Input: part model. Units: mm. Frame: model coordinates. Coordinates: 2 decimals unless noted, no trailing zeros. Write each loop counter-clockwise with the first axis right and the second up, starting at its lowest first coordinate (ties: lowest second). Pieces come first, ordered by that corner, then holes. Notation, with made-up numbers: (-17.5, 81) -> (22.5, 81) arc R27 ccw to (22.5, 119) -> close; hole circle Ø8 at (-26.5, -23). An arc over 180 degrees is marked (long way). One line per question, with ' | ' between items. Start each with the question number.
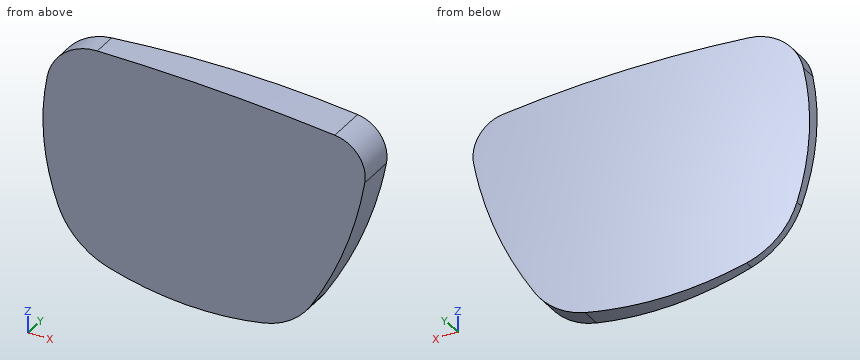
```python
from build123d import *

# Parameters (mm, degrees)
F1_DEPTH      = 25
F4_ANGLE_BACK = 15
F4_ANGLE      = 30


with BuildPart() as f1:
    # F0 (on Front) → F1 (new body)
    with BuildSketch(Plane.XZ):
        with BuildLine():
            ThreePointArc((26.3431364877, 8.5707053028), (25.1879544986, 13.2060879092), (21.0133194591, 15.5285089783))
            ThreePointArc((21.0133194591, 15.5285089783), (-0.0894086287, 17.0460813995), (-21.2428583947, 17.4457334904))
            ThreePointArc((-21.2428583947, 17.4457334904), (-27.0252643869, 15.3277245971), (-30.1521339791, 10.0225509634))
            ThreePointArc((-30.1521339791, 10.0225509634), (-30.737948683, -1.5598670025), (-28.1338702514, -12.8609448416))
            ThreePointArc((-28.1338702514, -12.8609448416), (-24.6579753008, -18.0246958087), (-19.2665178824, -21.1357015406))
            ThreePointArc((-19.2665178824, -21.1357015406), (-5.5690318774, -23.5254263951), (8.2977543738, -22.503591381))
            ThreePointArc((8.2977543738, -22.503591381), (13.1377213939, -20.4559972218), (16.7715565718, -16.6595298512))
            ThreePointArc((16.7715565718, -16.6595298512), (22.8064529235, -4.5182850542), (26.3431364877, 8.5707053028))
        make_face()
    extrude(amount=-F1_DEPTH)


with BuildPart() as f4:
    # F3 (on offset) → F4 (revolve)
    with BuildSketch(Plane.XY.offset(22), mode=Mode.PRIVATE) as f4_sk:
        with BuildLine():
            Line((-282, -293), (318, -293))
            ThreePointArc((318, -293), (18, 7), (-282, -293))
        make_face()
    revolve(f4_sk.sketch.rotate(Axis((18, -293, 22), (1, 0, 0)), -F4_ANGLE_BACK), axis=Axis((18, -293, 22), (1, 0, 0)), revolution_arc=F4_ANGLE)


with BuildPart() as f1_1:
    add(f1.part)

    # F5: intersect F4
    add(f4.part, mode=Mode.INTERSECT)


solid = f1_1.part
```
1) Section A-A, the plane y = 2.25. Return loops of the section in (x, z) (1 decimal).
2) Ray query, line 1 (Z direction, x = 20.5, y = 1.25); line 2 (Y direction, x = 2, z = 7); line 3 (Z direction, x = 18, y = 3.25). Return the intervals inside material, ascending.
3) First-contact query: P1, Ø6, axis at x = -24.5, z = -0.5, coming from the +Y side; P2, Ø4, axis at x = 6, y = 1, coming from the -Z side; P3, Ø1.5, axis at x = -24.5, z = -17, coming from the -Y side; P4, Ø1.5, axis at y = 2.5, z = 6, coming from the -X side. Flat tips, straight axial feed; report the tip coordinate or a pass-through.
4) Section B-B, the plane z = 14. Return loops of the section in (x, y), then the cut area to 3 significant figures.
5) Section C-C, the plane x = -16.5. Return loops of the section in (y, z).
Answer block:
1) outline: (-30.9, 1.1) arc R53.2 ccw to (-10.2, -23.1) arc R56.6 ccw to (8.3, -22.5) arc R13 ccw to (16.8, -16.7) arc R68.8 ccw to (26.3, 8.6) arc R6 ccw to (21, 15.5) arc R400 ccw to (-21.2, 17.4) arc R9.1 ccw to (-30.2, 10) arc R42 ccw to start
2) line 1: z = -9.9 to 15.58 | line 2: y = 0 to 6.2 | line 3: z = -14.62 to 15.81
3) P1: stops at y = 3.59 | P2: stops at z = -23.19 | P3: stops at y = 0 | P4: stops at x = -30.78
4) outline: (-28.32, 0) -> (24.46, 0) -> (24.46, 6.82) arc R299.89 ccw to (-28.32, 3.29) -> close | area: 308 mm2
5) outline: (0, -21.9) -> (1.76, -21.9) arc R298.01 ccw to (4.97, 17.45) -> (0, 17.45) -> close
